from build123d import *

# Parameters (mm, degrees)
F0_W     = 101.6
F0_H     = 45.72
F1_DEPTH = 101.6
F2_W     = 95.25
F2_H     = 95.25
F3_DEPTH = 44.45
F4_W     = 19.05
F4_H     = 6.35
F5_ANGLE = 180
F7_DEPTH = 25.4
F8_R     = 3.17499


# Not quite as in the source:
# - a fillet or chamfer is up to 0.001 mm smaller than in the source, because OpenCascade refuses the exact size


with BuildPart() as f1:
    # F0 (on Front) → F1 (new body)
    with BuildSketch(Plane.XZ):
        with Locations((17.3888143581, 4.6649015626)):
            Rectangle(F0_W, F0_H)
    extrude(amount=-F1_DEPTH)

    # F2 (on face) → F3 (cut)
    with BuildSketch(Plane.XY.offset(27.5249015626)):
        with Locations((17.3888143581, 50.8)):
            Rectangle(F2_W, F2_H)
    extrude(amount=-F3_DEPTH, mode=Mode.SUBTRACT)

    # F4 (on face) → F5 (revolve)
    with BuildSketch(Plane.XZ):
        with Locations((7.8638143581, 6.8874015626)):
            Rectangle(F4_W, F4_H)
        with Locations((7.8638143581, 0.5374015626)):
            Rectangle(F4_W, F4_H)
    revolve(axis=Axis((17.3888143581, 0, 3.7124015626), (0, 0, 1)), revolution_arc=F5_ANGLE)

    # F6 (on face) → F7 (cut)
    with BuildSketch(Plane.XY.offset(10.0624015626)):
        with BuildLine():
            Line((30.0888143581, 0), (4.6888143581, 0))
            ThreePointArc((4.6888143581, 0), (17.3888143581, -12.7), (30.0888143581, 0))
        make_face()
    extrude(amount=-F7_DEPTH, mode=Mode.SUBTRACT)

    # F8 (radius 3.175 in the source; OpenCascade refuses exactly that, so slightly less here)
    f8_edges = [f1.edges().sort_by_distance(p)[0] for p in [
        (17.388814, -19.05, 10.062402),
        (17.388814, -12.7, 10.062402),
        (17.388814, -19.05, -2.637598),
        (17.388814, -12.7, -2.637598),
    ]]
    fillet(f8_edges, radius=F8_R)


solid = f1.part
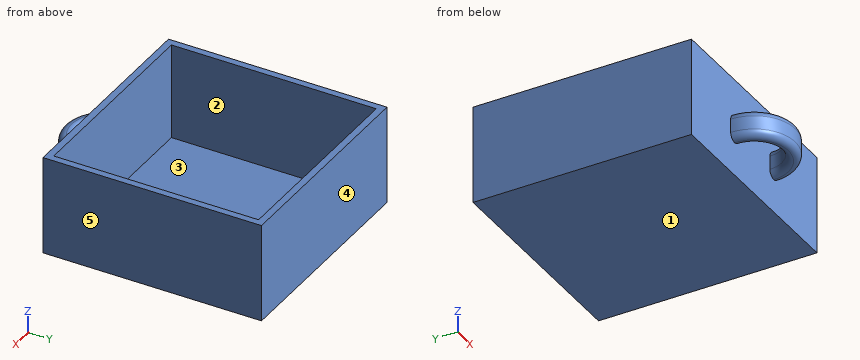
Work out the finished part from the listing and answer in its coordinate system (mm). Face numbers are marked on the shaded views. A direction names the side the tool comes from. Coordinates: 2 decimals unless noted, no trailing zeros. Loops run counter-clockwise (first coordinate to the right, second up) from the corner with the lowest first, then second, coordinate; pieces in that order, holes last. Notation, with made-up numbers: M -16,44.5 L 5,44.5 A35 cw 5,80.5 Z; hole C 53.25,-31 d1. An arc over 180 degrees is marked long. Answer in a Markdown table with one row per item. Add a question column.
1. The mould has two halves that part along Y. Classify the marked faces 3, 4 and 5: pulls with the +Y half, pulls with the -Y half, needs draft (parallel to the pull), parting line crosses it, or undercut.
2. Flat-ended cylindrical pins translate along their axes: P1, Ø4, axis at x = 23.5, y = 13.5, coming from the +Z side; P2, Ø12.5, axis at x = 17.5, y = -11, coming from the -Z side; P3, Ø1.5, axis at x = 38, z = -11, coming from the -Y side; P4, Ø12.5, axis at x = 23.5, y = -5.5, coming from the +Z side. Find the tip coordinate at first contact, or state that the pin passes through.
3. Consider L1, parallel to Y at x = 23, z = 22.5 (3 decimals); L2, parallel to X at y = 33.5, z = -5; L3, parallel to Y at x = 23, z = 0.5 (3 decimals). Determine where each line is inside the solid, lowest interval first.
4. Find section A-A, the plane z = 4.5. Write down the section's boundary in (x, y) (3 decimals).
5. A tool of negligible diameter and unlimited length cuts with its end or side. For the marked faces 1 and 2, from which of +Z, -Z, +X, -X, +Y, -Y can it reach the whole face along a straight path? Write none if from no direction.
6. Find section D-D, the plane x = 49.5. Write down the section's boundary in (y, z) (3 decimals), then the cut area to 3 significant figures.
7. Find section C-C, the plane y = 33.5. Write down the section's boundary in (x, z).
8. Find section B-B, the plane z = -7.5. Write down the section's boundary in (x, y) (3 decimals), then the cut area to 3 significant figures.
Reported:
| question | item | result |
|---|---|---|
| 1 | face 3 | undercut |
| 1 | face 4 | pulls with the +Y half |
| 1 | face 5 | needs draft |
| 2 | P1 | stops at z = -16.93 |
| 2 | P2 | stops at z = -2.64 |
| 2 | P3 | stops at y = 0 |
| 2 | P4 | stops at z = 27.52 |
| 3 | L1 | y = 0 to 3.175, 98.425 to 101.6 |
| 3 | L2 | x = -33.41 to -30.24, 65.01 to 68.19 |
| 3 | L3 | y = -18.205 to -11.393, 0 to 3.175, 98.425 to 101.6 |
| 4 | outline | M -33.411,0 L -1.661,0 A19.05 ccw 36.439,0 L 68.189,0 L 68.189,101.6 L -33.411,101.6 Z; hole M -30.236,3.175 L 65.014,3.175 L 65.014,98.425 L -30.236,98.425 Z; hole M 4.689,0 A12.7 ccw 30.089,0 Z |
| 5 | face 1 | -Z, +X, -X, +Y, -Y |
| 5 | face 2 | +Z |
| 6 | outline | M 0,-18.195 L 101.6,-18.195 L 101.6,27.525 L 98.425,27.525 L 98.425,-16.925 L 3.175,-16.925 L 3.175,27.525 L 0,27.525 Z |
| 6 | area | 411 mm^2 |
| 7 | outline | M -33.41,-18.2 L 68.19,-18.2 L 68.19,27.52 L 65.01,27.52 L 65.01,-16.93 L -30.24,-16.93 L -30.24,27.52 L -33.41,27.52 Z |
| 8 | outline | M -33.411,0 L 68.189,0 L 68.189,101.6 L -33.411,101.6 Z; hole M -30.236,3.175 L 65.014,3.175 L 65.014,98.425 L -30.236,98.425 Z |
| 8 | area | 1,250 mm^2 |
